```python
from build123d import *

# Parameters (mm, degrees)
SKETCH_1_R          = 3.405
EXTRUDE_1_DEPTH     = 4.5
EXTRUDE_2_DEPTH     = 1.52
SKETCH_3_R          = 0.5
CUT_EXTRUDE_1_DEPTH = 1.52


with BuildPart() as part:
    # 草图1 → 凸台-拉伸1 (new body)
    with BuildSketch(Plane(origin=(0, 0, 0), x_dir=(1, 0, 0), z_dir=(0, 1, 0))):
        Circle(SKETCH_1_R)
    extrude(amount=EXTRUDE_1_DEPTH)

    # 草图2 → 凸台-拉伸2 (add)
    with BuildSketch(Plane.XZ):
        with BuildLine():
            Line((2.314339904, 2.497569981), (13.854119989, 1.847067684))
            ThreePointArc((13.854119989, 1.847067684), (15.6, 0), (13.854119989, -1.847067684))
            Line((13.854119989, -1.847067684), (2.314339904, -2.497569981))
            ThreePointArc((2.314339904, -2.497569981), (0, -3.405), (-2.314339904, -2.497569981))
            Line((-2.314339904, -2.497569981), (-13.854119989, -1.847067684))
            ThreePointArc((-13.854119989, -1.847067684), (-15.6, 0), (-13.854119989, 1.847067684))
            Line((-13.854119989, 1.847067684), (-2.314339904, 2.497569981))
            ThreePointArc((-2.314339904, 2.497569981), (0, 3.405), (2.314339904, 2.497569981))
        make_face()
    extrude(amount=-EXTRUDE_2_DEPTH)

    # 草图3 → 切除-拉伸1 (cut)
    with BuildSketch(Plane.XZ):
        with Locations((4, 0)):
            Circle(SKETCH_3_R)
        with Locations((5.8, 0)):
            Circle(SKETCH_3_R)
        with Locations((7.6, 0)):
            Circle(SKETCH_3_R)
        with Locations((9.4, 0)):
            Circle(SKETCH_3_R)
        with Locations((11.2, 0)):
            Circle(SKETCH_3_R)
        with Locations((13, 0)):
            Circle(SKETCH_3_R)
        with Locations((14.8, 0)):
            Circle(SKETCH_3_R)
    extrude(amount=-CUT_EXTRUDE_1_DEPTH, mode=Mode.SUBTRACT)


solid = part.part
```
Model file for the job. Use its own axes, mm. Coordinates: 2 decimals unless noted, no trailing zeros. Loops run counter-clockwise (first coordinate to the right, second up) from the corner with the lowest first, then second, coordinate; pieces in that order, holes last. Notation, with made-up numbers: (-24, -17.75) - (-13, -17.75) arc R19 ccw to (-13, 4.25) - close; hole circle Ø5 at (-21.5, -2). An arc over 180 degrees is marked (long way). Write item = value, one per line. Start each with the question number.
Item 1: Saw through at B-B, the plane x = 7.6. List the corners of the cut face in (y, z).
Item 2: Saw through at D-D, the plane x = 11.2. List the corners of the cut face in (y, z), then the cut area to 3 significant figures.
Item 3: Saw through at A-A, the plane y = 1.15. List the corners of the cut face in (x, z) (3 decimals).
Item 4: Wall check: probe 1 along Y at (x, z) = (5, 1.75); probe 2 along Z at (x, y) = (5.8, 0.85); probe 3 along Z at (x, y) = (11.2, 0.7). Give the ranges that are in metal, low to high. Write a range as [from, to].
Item 5: Saw through at C-C, the plane z = -1. List the corners of the cut face in (x, y), then the cut area to 3 significant figures.
Item 6: Drop flat-ended pins along their axis: pin 1 Ø1.5 at (x, z) = (-9, 0.5) entering from +Y; pin 2 Ø1.5 at (y, z) = (2.5, -0.5) entering from -X (3 decimals). Give the stop position or say it passes through.
Item 7: Pull direction X, two halves, no side cores. Call faces 1 (the face through (-8.165, 0.749, 2.168)), 2 (the face through (15.6, 0.7, 0)), 3 (the face through (-9, 1.52, 0)), 4 (the face through (9.862, 0.749, -0.192)): +X half, -X half, draft (parallel to the pull), parting line (faces both ways), or undercut.
Answers:
q1.outline = (0, -2.2) - (1.52, -2.2) - (1.52, -0.5) - (0, -0.5) - close; (0, 0.5) - (1.52, 0.5) - (1.52, 2.2) - (0, 2.2) - close
q2.outline = (0, -2) - (1.52, -2) - (1.52, -0.5) - (0, -0.5) - close; (0, 0.5) - (1.52, 0.5) - (1.52, 2) - (0, 2) - close
q2.area = 4.55 mm2
q3.outline = (-13.854, -1.847) - (-2.314, -2.498) arc R3.405 ccw to (2.314, -2.498) - (13.854, -1.847) arc R1.85 ccw to (13.854, 1.847) - (2.314, 2.498) arc R3.405 ccw to (-2.314, 2.498) - (-13.854, 1.847) arc R1.85 ccw to start; hole circle Ø1 at (4, 0); hole circle Ø1 at (5.8, 0); hole circle Ø1 at (7.6, 0); hole circle Ø1 at (9.4, 0); hole circle Ø1 at (11.2, 0); hole circle Ø1 at (13, 0); hole circle Ø1 at (14.8, 0)
q4.probe_1 = [0, 1.52]
q4.probe_2 = [-2.3, -0.5], [0.5, 2.3]
q4.probe_3 = [-2, -0.5], [0.5, 2]
q5.outline = (-15.31, 0) - (15.31, 0) - (15.31, 1.52) - (3.25, 1.52) - (3.25, 4.5) - (-3.25, 4.5) - (-3.25, 1.52) - (-15.31, 1.52) - close
q5.area = 65.9 mm2
q6.pin_1 = 1.52
q6.pin_2 = -3.405
q7.face_1 = -X half
q7.face_2 = +X half
q7.face_3 = draft
q7.face_4 = undercut
